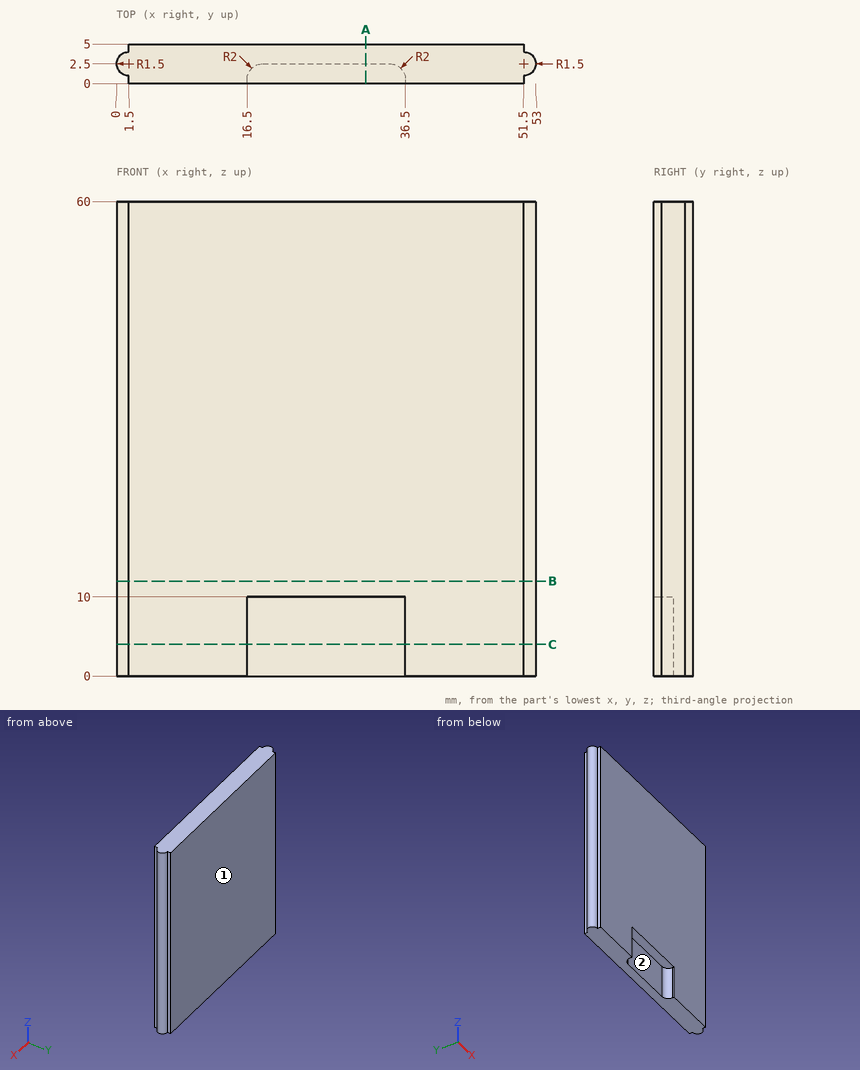
Input: dimensioned drawing with shaded views. Units: mm. Origin: part minimum x, y, z. A direction names the side the tool comes from. Give positions to 0.01 mm unless a question says otherwise; leave off trailing zeros. Write each loop counter-clockwise with the first axis right and the second up, starting at its lowest first coordinate (ties: lowest second). Pieces come first, ordered by that corner, then holes. Notation, with made-up numbers: (9.5, 2) -> (13.5, 2) arc R19 cw to (13.5, 38) -> close; hole circle Ø4 at (38.25, 0). An arc over 180 degrees is marked (long way). Answer as a JSON object with one key per item and string values.
1. Cut plane B-B on z = 12. Output: boundary loops of the cut face in (x, y), and give its area (3 significant figures).
Ans:
{"outline": "(1.5, 0) -> (51.5, 0) -> (51.5, 1) arc R1.5 ccw to (51.5, 4) -> (51.5, 5) -> (1.5, 5) -> (1.5, 4) arc R1.5 ccw to (1.5, 1) -> close", "area": "257 mm^2"}
2. Cut plane A-A on x = 31.5. Output: boundary loops of the cut face in (y, z).
Ans:
{"outline": "(0, 10) -> (2.5, 10) -> (2.5, 0) -> (5, 0) -> (5, 60) -> (0, 60) -> close"}
3. Ray query, probe 1 along X at (y, z) = (2.65, 27); probe 2 along X at (y, z) = (0.4, 33); probe 3 along Z at (x, y) = (22.5, 0.5). Return the intervals inside material, ascending. Write a range as from..to.
Ans:
{"probe 1": "x = 0.01..52.99", "probe 2": "x = 1.5..51.5", "probe 3": "z = 10..60"}
4. Access query for the marked faces 1 and 2. Directions: +Z, -Z, +X, -X, +Y, -Y. A direction counts if a zero-diameter tool reaches every point of the face in a straight line with its end or side. Return the directions, or none.
Ans:
{"face 1": "+Z, -Z, +X, -X, +Y", "face 2": "-Z, -Y"}
5. Contact query for flat-ended pins moving along their axis: pin 1 (2 mm diameter, centred on x = 26, y = 1, fed in from -Z); pin 2 (3 mm diameter, centred on y = 4.5, z = 22.5, fed in from -X); pin 3 (0.5 mm diameter, centred on y = 4.5, z = 40, fed in from -X). Output: stop coordinate, or through.
Ans:
{"pin 1": "stops at z = 10", "pin 2": "stops at x = 0.09", "pin 3": "stops at x = 1.5"}
6. Cut plane C-C on z = 4. Output: boundary loops of the cut face in (x, y).
Ans:
{"outline": "(1.5, 0) -> (16.5, 0) -> (16.5, 0.5) arc R2 cw to (18.5, 2.5) -> (34.5, 2.5) arc R2 cw to (36.5, 0.5) -> (36.5, 0) -> (51.5, 0) -> (51.5, 1) arc R1.5 ccw to (51.5, 4) -> (51.5, 5) -> (1.5, 5) -> (1.5, 4) arc R1.5 ccw to (1.5, 1) -> close"}
